Geometry: final body of the model. Coordinates: model frame, mm. Face numbers are marked on the shaded views. A direction names the side the tool comes from. Give positions to 0.01 mm unless a question says otherwise; leave off trailing zeros. Write each loop counter-clockwise with the first axis right and the second up, starting at its lowest first coordinate (ties: lowest second). Pieces come first, ordered by that corner, then holes. Notation, with made-up numbers: (50, 23.5) -> (102, 23.5) arc R22 cw to (102, 60.5) -> close; hole circle Ø6 at (35, 56). An arc over 180 degrees is marked (long way). Answer in a Markdown table with one row per item. Add a question column.
Item 1: Section query A-A on y = 0. Output: boundary loops of the cut face in (x, z).
Item 2: Draft query along Y for the marked faces 1, 2 and 3. Return one class per face: +Y half, -Y half, draft (parallel to the pull), parting line (faces both ways), or undercut.
Item 3: Section query B-B on z = -7. Output: boundary loops of the cut face in (x, y).
Item 4: Material intervals for probe 1 along X at (y, z) = (0, -7.5); probe 2 along Z at (x, y) = (2.5, 0.5), sorted ascending. Write a range as from..to.
Item 5: Access query for the marked faces 4 and 5. Directions: +Z, -Z, +X, -X, +Y, -Y. A direction counts if a zero-diameter tool reaches every point of the face in a straight line with its end or side. Return the directions, or none.
Item 6: First-contact query: P1, Ø5, axis at x = -2, z = -8.5, coming from the +Y side; P2, Ø4, axis at y = 2, z = -1, coming from the -X side; P3, Ø2, axis at x = 2.5, z = -11.5, coming from the -Y side; P4, Ø1, axis at x = -1, y = -2, coming from the -Z side. Flat tips, straight axial feed; report the tip coordinate or a pass-through.
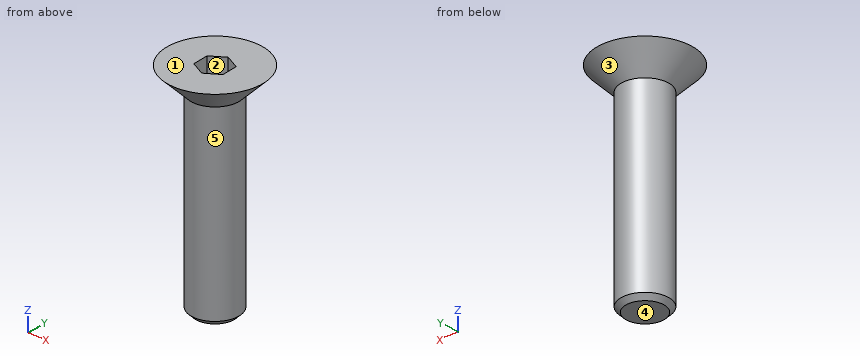
```python
from build123d import *

# Parameters (mm, degrees)
F0_R        = 5
F1_DEPTH    = 2.7
F4_DEPTH    = 2
F2_R        = 2.5
F5_DEPTH    = 20
F6_SIZE     = 0.5
F7_S5_R     = 2.5
F7_T6_DEPTH = 9


# Not quite as in the source:
# - a fillet or chamfer that OpenCascade refuses, or shapes differently, is made with other operations: its cross-section is extruded or revolved along the edge and cut away or added
# - a feature names something its author has since deleted; it is built from what else it names


with BuildPart() as f1:
    # F0 (on Top) → F1 (new body)
    with BuildSketch(Plane.XY):
        Circle(F0_R)
    extrude(amount=F1_DEPTH)

    # F3 (on face) → F4 (cut)
    with BuildSketch(Plane.XY.offset(2.7)):
        Polygon((1.4221256636, 0.98871563), (-0.1451900209, 1.725954767), (-1.5673156845, 0.737239137), (-1.4221256636, -0.98871563), (0.1451900209, -1.725954767), (1.5673156845, -0.737239137), align=None)
    extrude(amount=-F4_DEPTH, mode=Mode.SUBTRACT)

    # F2 (on face) → F5 (join)
    with BuildSketch(Plane(origin=(0, 0, 0), x_dir=(1, 0, 0), z_dir=(0, 0, -1))):
        Circle(F2_R)
    extrude(amount=F5_DEPTH)

    # F6
    f6_edges = [f1.edges().sort_by_distance(p)[0] for p in [
        (-2.5, 0, -20),
    ]]
    chamfer(f6_edges, length=F6_SIZE)

    # F7: chamfer of 2.7 on 1 edges, made by hand


with BuildPart() as f7_tool2:
    # F7_s3 → F7_t4 (revolve)
    with BuildSketch(Plane.XZ):
        Polygon((2.3, 0), (5, 2.7), (5, 0), align=None)
    revolve(axis=Axis((0, 0, 0), (0, 0, 1)))

    # F7_s5 → F7_t6 (cut, symmetric)
    with BuildSketch(Plane.XY.offset(1.4)):
        Circle(F7_S5_R)
    extrude(amount=F7_T6_DEPTH, both=True, mode=Mode.SUBTRACT)


with BuildPart() as f1_1:
    add(f1.part)

    # F7_t1: cut F7_tool2
    add(f7_tool2.part, mode=Mode.SUBTRACT)


solid = f1_1.part
```
Findings below:
| question | item | result |
|---|---|---|
| 1 | outline | (-5, 2.7) -> (-2.5, 0.2) -> (-2.5, -19.5) -> (-2, -20) -> (2, -20) -> (2.5, -19.5) -> (2.5, 0.2) -> (5, 2.7) -> (1.51, 2.7) -> (1.51, 0.7) -> (-1.51, 0.7) -> (-1.51, 2.7) -> close |
| 2 | face 1 | draft |
| 2 | face 2 | undercut |
| 2 | face 3 | parting line |
| 3 | outline | circle Ø5 at (0, 0) |
| 4 | probe 1 | x = -2.5..2.5 |
| 4 | probe 2 | z = 0.25..2.7 |
| 5 | face 4 | -Z, +X, -X, +Y, -Y |
| 5 | face 5 | -Z |
| 6 | P1 | stops at y = 2.5 |
| 6 | P2 | stops at x = -2.9 |
| 6 | P3 | stops at y = -2 |
| 6 | P4 | stops at z = -20 |
